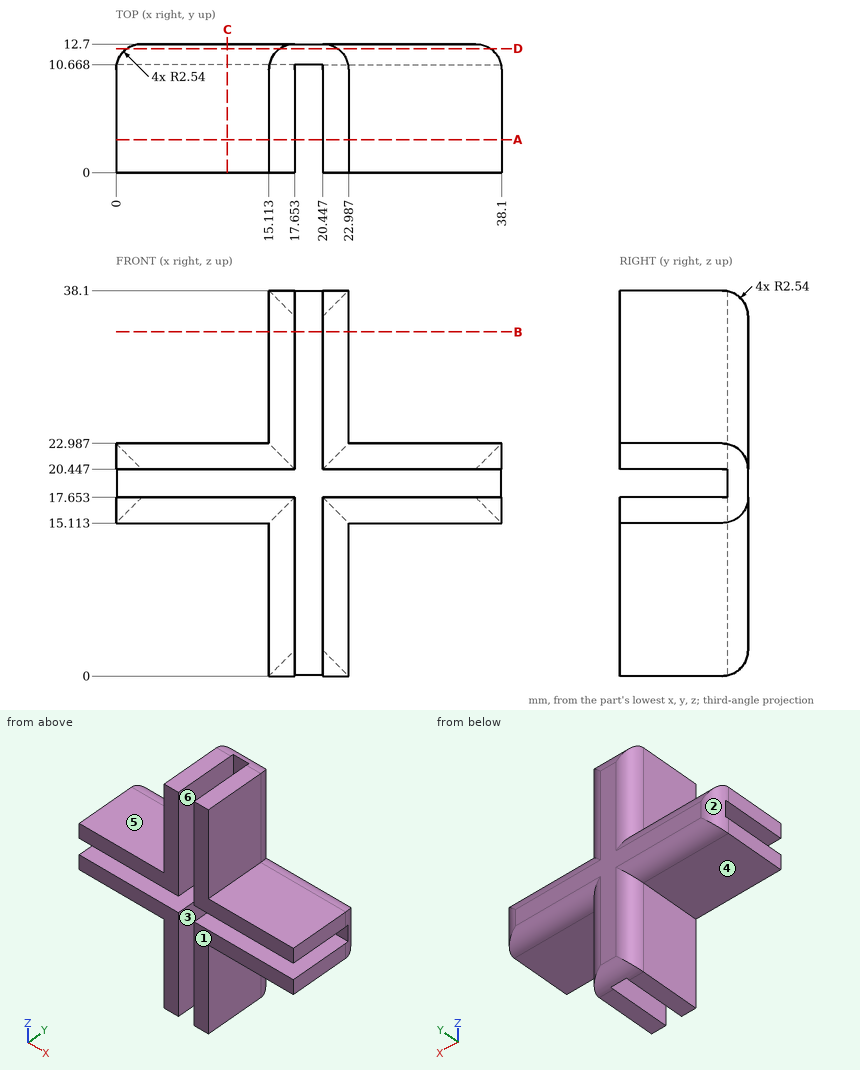
Source: three-view drawing plus pictorial views. Frame: mm from the lowest corner of the part. A direction names the side the tool comes from. Coordinates: 2 decimals unless noted, no trailing zeros. Order: outer loops, then holes, each group sorted by start corner. A loop starts at its lowest first (then second) coordinate and runs counter-clockwise, first axis right, second up. Notation, with made-up numbers: (17, 60.5) -> (25, 60.5) arc R32 ccw to (25, 90.5) -> close; hole circle Ø11 at (49.25, 88.25). An arc over 180 degrees is marked (long way). Write item = value, one per line.
(1) Access query for the marked faces 4, 5 and 6. Directions: +Z, -Z, +X, -X, +Y, -Y. A direction counts if a zero-diameter tool reaches every point of the face in a straight line with its end or side. Return the directions, or none.
Solved:
face_4 = -Z, -X, +Y, -Y
face_5 = +Z, -X, +Y, -Y
face_6 = +Z, -Z, -Y
(2) Cut plane C-C on x = 11. Return loops of the section in (y, z).
Solved:
outline = (0, 15.11) -> (10.16, 15.11) arc R2.54 ccw to (12.7, 17.65) -> (12.7, 20.45) arc R2.54 ccw to (10.16, 22.99) -> (0, 22.99) -> (0, 20.45) -> (10.67, 20.45) -> (10.67, 17.65) -> (0, 17.65) -> close
(3) Cut plane D-D on y = 12.25. Return loops of the section in (x, z).
Solved:
outline = (1.1, 16.21) -> (16.21, 16.21) -> (16.21, 1.1) -> (21.89, 1.1) -> (21.89, 16.21) -> (37, 16.21) -> (37, 21.89) -> (21.89, 21.89) -> (21.89, 37) -> (16.21, 37) -> (16.21, 21.89) -> (1.1, 21.89) -> close
(4) Line query: line 1 (Z direction, x = 25.5, y = 2.75); line 2 (Z direction, x = 22, y = 10). Output: solid intervals per line, ascending.
Solved:
line_1 = 15.11 to 17.65, 20.45 to 22.99
line_2 = 0 to 17.65, 20.45 to 38.1
(5) Pull-direction query (X, two-part tool) for the marked faces 1, 2 and 3; classes: pulls with the +X half, pulls with the -X half, needs draft (parallel to the pull), parting line crosses it, or undercut.
Solved:
face_1 = needs draft
face_2 = pulls with the -X half
face_3 = undercut
(6) Cut plane A-A on y = 3.25. Return loops of the section in (x, z).
Solved:
outline = (0, 15.11) -> (15.11, 15.11) -> (15.11, 0) -> (17.65, 0) -> (17.65, 17.65) -> (0, 17.65) -> close; (0, 20.45) -> (17.65, 20.45) -> (17.65, 38.1) -> (15.11, 38.1) -> (15.11, 22.99) -> (0, 22.99) -> close; (20.45, 0) -> (22.99, 0) -> (22.99, 15.11) -> (38.1, 15.11) -> (38.1, 17.65) -> (20.45, 17.65) -> close; (20.45, 20.45) -> (38.1, 20.45) -> (38.1, 22.99) -> (22.99, 22.99) -> (22.99, 38.1) -> (20.45, 38.1) -> close
(7) Cut plane B-B on z = 34. Return loops of the section in (x, y).
Solved:
outline = (15.11, 0) -> (17.65, 0) -> (17.65, 10.67) -> (20.45, 10.67) -> (20.45, 0) -> (22.99, 0) -> (22.99, 10.16) arc R2.54 ccw to (20.45, 12.7) -> (17.65, 12.7) arc R2.54 ccw to (15.11, 10.16) -> close
(8) Pin query (flat end, axial travel): pin 1 Ø5.5 at (x, y) = (26, 6.5) entering from -Z; pin 2 Ø5.5 at (x, y) = (8, 5.5) entering from +Z; pin 3 Ø4 at (y, z) = (6.5, 8) entering from +X. Return the tip coordinate at first contact, or that it passes through.
Solved:
pin_1 = 15.11
pin_2 = 22.99
pin_3 = 22.99
